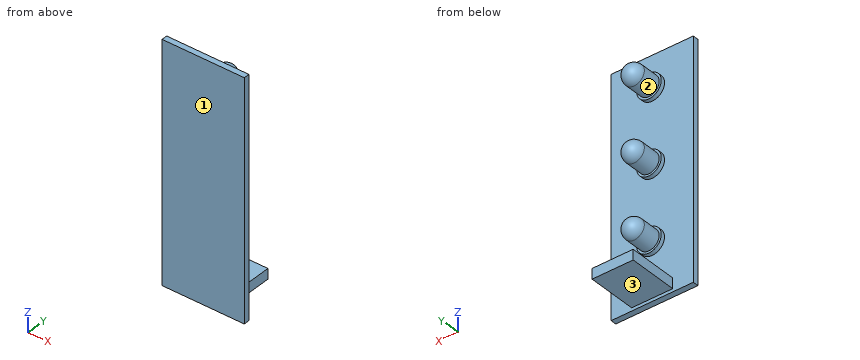
Autodesk Inventor part; units mm, degrees
ref_plane "YZ Plane" through (0, 0, 0) normal (1, 0, 0) x (0, 1, 0)
ref_plane "XZ Plane" through (0, 0, 0) normal (0, 1, 0) x (-1, 0, 0)
ref_plane "XY Plane" through (0, 0, 0) normal (0, 0, 1) x (1, 0, 0)
sketch "Sketch1" plane through (0, 0, 0) normal (0, 1, 0) x (-1, 0, 0)
  line L0 (20, 0) -> (0, 0)
  line L1 (0, 0) -> (0, -57.5)
  line L2 (0, -57.5) -> (20, -57.5)
  line L3 (20, -57.5) -> (20, 0)
  circle A0 centre (10, -7.75) radius 2.5
  circle A1 centre (10, -25.75) radius 2.5
  circle A2 centre (10, -43.75) radius 2.5
  line L4 (15, -54.25) -> (5, -54.25)
  line L5 (5, -54.25) -> (5, -56.75)
  line L6 (5, -56.75) -> (15, -56.75)
  line L7 (15, -56.75) -> (15, -54.25)
  circle A3 centre (10, -7.75) radius 3
  circle A4 centre (10, -25.75) radius 3
  circle A5 centre (10, -43.75) radius 3
  dimension "d0" = 57.5
  dimension "d1" = 20
  dimension "d2" = 5
  dimension "d3" = 5
  dimension "d4" = 5
  dimension "d8" = 0.75
  dimension "d9" = 2.5
  dimension "d10" = 10
  dimension "d20" = 10
  dimension "d21" = 5
  dimension "d22" = 6
  dimension "d23" = 6
  dimension "d24" = 6
  dimension "d45" = 7.75
  dimension "d46" = 18
  dimension "d47" = 18
extrude "Extrusion1" add sketch "Sketch1" against normal blind 1.4 contours L3 L2 L1 L0 | A0 | A1 | A2 | L7 L6 L5 L4 | A3 | A4 | A5
extrude "Extrusion2" add sketch "Sketch1" along normal blind 12 contours L7 L6 L5 L4
extrude "Extrusion5" add sketch "Sketch1" along normal blind 8 contours A0
extrude "Extrusion6" add sketch "Sketch1" along normal blind 1 contours A3
fillet "Fillet4" radius 2.5 1 edges at (-7.5, 8, -7.75)
extrude "Extrusion7" add sketch "Sketch1" along normal blind 1 contours A4
extrude "Extrusion8" add sketch "Sketch1" along normal blind 8 contours A1
fillet "Fillet5" radius 2.5 1 edges at (-7.5, 8, -25.75)
extrude "Extrusion9" add sketch "Sketch1" along normal blind 8 contours A2
extrude "Extrusion10" add sketch "Sketch1" along normal blind 1 contours A5
fillet "Fillet6" radius 2.5 1 edges at (-7.5, 8, -43.75)
properties part number "Led_Board_V1"
Input: part model. Units: mm. Frame: model coordinates. Face numbers are marked on the shaded views. Give positions to 0.01 mm unless a question says otherwise; leave off trailing zeros. Order: outer loops, then holes, each group sorted by start corner. A loop starts at its lowest first (then second) coordinate and runs counter-clockwise, first axis right, second up.
Q1. Section D-D on y = 9. Output: boundary loops of the cut face in (x, z).
Checked values:
outline: (-15, -56.75) - (-5, -56.75) - (-5, -54.25) - (-15, -54.25) - close
Q2. Draft query along Z for the marked faces 1, 2 and 3. Return one class per face: +Z half, -Z half, draft (parallel to the pull), parting line (faces both ways), or undercut.
Checked values:
face 1: draft
face 2: undercut
face 3: -Z half
Q3. Section A-A on z = -7.75. Output: boundary loops of the cut face in (x, y), and give its area (3 significant figures).
Checked values:
outline: (-20, -1.4) - (0, -1.4) - (0, 0) - (-7, 0) - (-7, 1) - (-7.5, 1) - (-7.5, 5.5) arc R2.5 ccw to (-12.5, 5.5) - (-12.5, 1) - (-13, 1) - (-13, 0) - (-20, 0) - close
area: 66.3 mm2
Q4. Ray query, probe 1 along Z at (x, y) = (-9, 2.5); probe 2 along Z at (x, y) = (-8, 5.5); probe 3 along Y at (x, z) = (-9.5, -48). Return the intervals inside material, ascending.
Checked values:
probe 1: z = -56.75 to -54.25, -46.04 to -41.46, -28.04 to -23.46, -10.04 to -5.46
probe 2: z = -56.75 to -54.25, -45.25 to -42.25, -27.25 to -24.25, -9.25 to -6.25
probe 3: y = -1.4 to 0
Q5. Section C-C on y = 6.5. Output: boundary loops of the cut face in (x, z).
Checked values:
outline: (-15, -56.75) - (-5, -56.75) - (-5, -54.25) - (-15, -54.25) - close; circle Ø4.58 at (-10, -43.75); circle Ø4.58 at (-10, -25.75); circle Ø4.58 at (-10, -7.75)
Q6. Contact query for flat-ended pins moving along their axis: pin 1 Ø6 at (x, z) = (-7.5, -17.5) entering from +Y; pin 2 Ø3 at (y, z) = (8, -55.5) entering from +X; pin 3 Ø12 at (x, z) = (-12.5, -39.5) entering from +Y. Output: stop coordinate, or through.
Checked values:
pin 1: stops at y = 0
pin 2: stops at x = -5
pin 3: stops at y = 8
